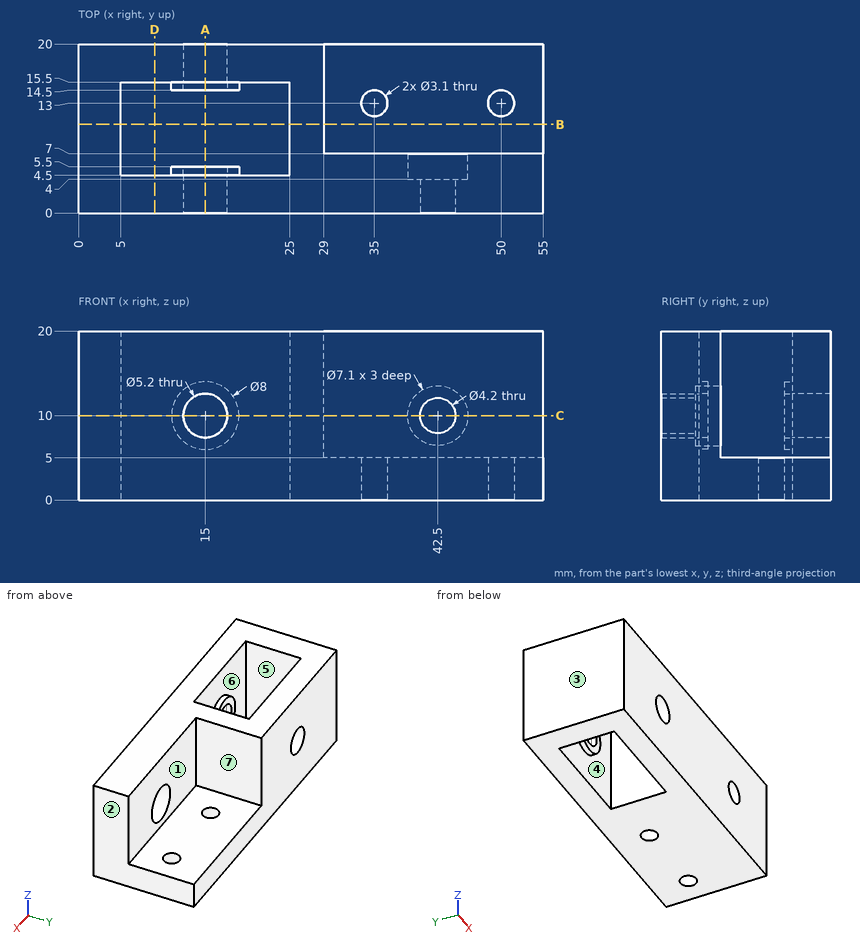
Can you work these out from the drawing? Everything is in mm from the part's minimum corner. A direction names the side the tool comes from. Round coordinates to 2 decimals unless told otherwise and drop trailing zeros. Loops run counter-clockwise (first coordinate to the right, second up) from the corner with the lowest first, then second, coordinate; pieces in that order, holes last. Notation, with made-up numbers: (87.25, 49.5) -> (99.25, 49.5) arc R21 ccw to (99.25, 80.5) -> close; hole circle Ø5 at (21.5, 13.5). An arc over 180 degrees is marked (long way). Use CSV: the item, a comma, the result in double quotes.
(1) Suppose I cut it at A-A on x = 15. Write out the boundary of the cut face in (y, z), plus the area to 3 significant figures.
Return value:
outline,"(0, 0) -> (4.5, 0) -> (4.5, 6) -> (5.5, 6) -> (5.5, 7.4) -> (0, 7.4) -> close; (0, 12.6) -> (5.5, 12.6) -> (5.5, 14) -> (4.5, 14) -> (4.5, 20) -> (0, 20) -> close; (14.5, 6) -> (15.5, 6) -> (15.5, 0) -> (20, 0) -> (20, 7.4) -> (14.5, 7.4) -> close; (14.5, 12.6) -> (20, 12.6) -> (20, 20) -> (15.5, 20) -> (15.5, 14) -> (14.5, 14) -> close"
area,"139 mm²"
(2) Suppose I cut it at C-C on z = 10. Give the number of separate pieces and of enclosed holes in the cut face, plus the area to 3 significant figures.
Return value:
separate pieces,"3"
enclosed holes,"0"
area,"463 mm²"
(3) If we mould it in two halves opening along X, with no side actions, what happens to the marked faces 1, 2, 3 and 4? For each: +X half, -X half, draft (parallel to the pull), parting line (faces both ways), or undercut.
Return value:
face 1,"draft"
face 2,"+X half"
face 3,"-X half"
face 4,"undercut"
(4) For the marked faces 5, 6 and 7, which set-ups out of +Z, -Z, +X, -X, +Y, -Y let a thin tool reach every point of the face, with its end or its side?
Return value:
face 5,"+Z, -Z"
face 6,"none"
face 7,"+Z, +X, +Y"
(5) If I drill on probe 1 along X at (y, z) = (13, 2.95); probe 2 along X at (y, z) = (8.5, 9); probe 3 along Z at (x, y) = (42.5, 5.15), over which ranges is the centre line in solid material (lowest first)? Write a range as [from, to].
Return value:
probe 1,"x = [0, 5], [25, 33.45], [36.55, 48.45], [51.55, 55]"
probe 2,"x = [0, 5], [25, 29]"
probe 3,"z = [0, 6.45], [13.55, 20]"
(6) Suppose I cut it at B-B on y = 10.5. Write out the boundary of the cut face in (x, z), plus the area to 3 significant figures.
Return value:
outline,"(0, 0) -> (5, 0) -> (5, 20) -> (0, 20) -> close; (25, 0) -> (55, 0) -> (55, 5) -> (29, 5) -> (29, 20) -> (25, 20) -> close"
area,"310 mm²"
(7) Suppose I cut it at D-D on x = 9. Write out the boundary of the cut face in (y, z), plus the area to 3 significant figures.
Return value:
outline,"(0, 0) -> (4.5, 0) -> (4.5, 20) -> (0, 20) -> close; (15.5, 0) -> (20, 0) -> (20, 20) -> (15.5, 20) -> close"
area,"180 mm²"
(8) Will these pins go through, and if not, where does the flat tip stop? pin 1 Ø2 at (x, z) = (43.5, 11.5) entering from +Y; pin 2 Ø8 at (x, z) = (42.5, 10) entering from +Y; pin 3 Ø6 at (y, z) = (10.5, 17) entering from +X.
Return value:
pin 1,"stops at y = 4"
pin 2,"stops at y = 7"
pin 3,"stops at x = 29"
